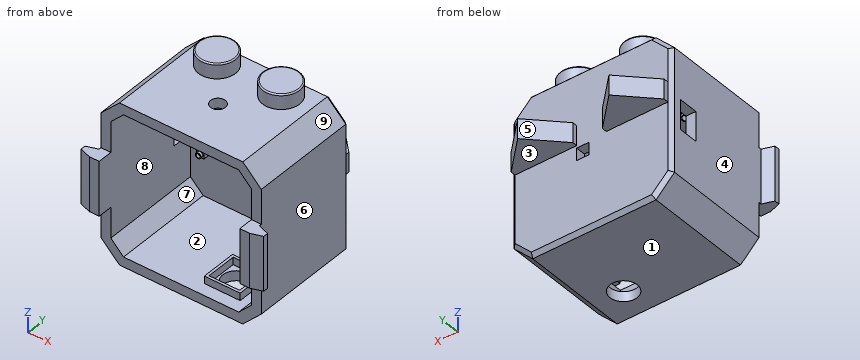
from build123d import *

# Parameters (mm, degrees)
SALIENTE_EXTRUIR1_DEPTH  = 45
VACIADO2_T               = -4
CHAFL_N3_SIZE            = 1.5
CROQUIS2_R               = 7.5
SALIENTE_EXTRUIR2_DEPTH  = 6
CROQUIS4_R               = 5
CORTAR_EXTRUIR2_DEPTH    = 8
REDONDEO1_R              = 0.5
CROQUIS5_R               = 3
CORTAR_EXTRUIR3_DEPTH    = 10
SALIENTE_EXTRUIR8_START  = 8
CROQUIS13_R              = 5
CROQUIS13_R_2            = 2.6
SALIENTE_EXTRUIR8_DEPTH  = 8
CROQUIS7_W               = 4
CROQUIS7_H               = 4
SALIENTE_EXTRUIR3_DEPTH  = 1
CROQUIS8_R               = 2
SALIENTE_EXTRUIR4_DEPTH  = 1
CROQUIS9_R               = 1.6
CORTAR_EXTRUIR5_DEPTH    = 2
CROQUIS10_W              = 25
CROQUIS10_H              = 8
SALIENTE_EXTRUIR5_DEPTH  = 2
SALIENTE_EXTRUIR6_DEPTH  = 8
CROQUIS12_R              = 1.15
CROQUIS12_R_2            = 0.8
SALIENTE_EXTRUIR7_DEPTH  = 6
CROQUIS14_W              = 3
CROQUIS14_H              = 2.5
SALIENTE_EXTRUIR9_DEPTH  = 5
CROQUIS15_W              = 12
CROQUIS15_H              = 8
CORTAR_EXTRUIR6_DEPTH    = 7
CROQUIS16_W              = 14.5
CROQUIS16_H              = 14.5
CROQUIS16_W_2            = 12.4
CROQUIS16_H_2            = 12.4
SALIENTE_EXTRUIR10_DEPTH = 3
CROQUIS17_R              = 5.5
CORTAR_EXTRUIR7_DEPTH    = 96.317889192
CROQUIS18_W              = 4
CROQUIS18_H              = 22
SALIENTE_EXTRUIR11_DEPTH = 6
SALIENTE_EXTRUIR13_DEPTH = 22
CROQUIS20_W              = 5
CROQUIS20_H              = 5
CORTAR_EXTRUIR8_DEPTH    = 10


with BuildPart() as part:
    # Croquis1 → Saliente-Extruir1 (new body)
    with BuildSketch(Plane(origin=(0, 0, 0), x_dir=(1, 0, 0), z_dir=(0, 1, 0))):
        Polygon((-25, -32.5), (25, -32.5), (32.5, -25), (32.5, 25), (25, 32.5), (-25, 32.5), (-32.5, 25), (-32.5, -25), align=None)
    extrude(amount=SALIENTE_EXTRUIR1_DEPTH)

    # Vaciado2
    vaciado2_openings = [part.faces().sort_by_distance(p)[0] for p in [
        (0, 0, 0),
    ]]
    offset(amount=VACIADO2_T, openings=vaciado2_openings, kind=Kind.INTERSECTION)

    # Chaflán3
    chafl_n3_edges = [part.edges().sort_by_distance(p)[0] for p in [
        (-28.75, 45, -28.75),
        (-32.5, 45, 0),
        (-28.75, 45, 28.75),
        (0, 45, 32.5),
        (28.75, 45, 28.75),
        (32.5, 45, 0),
        (28.75, 45, -28.75),
        (0, 45, -32.5),
    ]]
    chamfer(chafl_n3_edges, length=CHAFL_N3_SIZE)

    # Croquis2 → Saliente-Extruir2 (add)
    with BuildSketch(Plane.XY.offset(32.5)):
        with Locations(Location((13, 35, 0), (0, 0, 180))):
            Circle(CROQUIS2_R)
        with Locations(Location((-13, 35, 0), (0, 0, 180))):
            Circle(CROQUIS2_R)
    extrude(amount=SALIENTE_EXTRUIR2_DEPTH)

    # Croquis4 → Cortar-Extruir2 (cut)
    with BuildSketch(Plane(origin=(0, 0, 28.5), x_dir=(-1, 0, 0), z_dir=(0, 0, -1))):
        with Locations((-13, 35)):
            Circle(CROQUIS4_R)
        with Locations(Location((13, 35, 0), (0, 0, 180))):
            Circle(CROQUIS4_R)
    extrude(amount=-CORTAR_EXTRUIR2_DEPTH, mode=Mode.SUBTRACT)

    # Redondeo1
    redondeo1_edges = [part.edges().sort_by_distance(p)[0] for p in [
        (20.5, 35, 38.5),
        (-5.5, 35, 38.5),
    ]]
    fillet(redondeo1_edges, radius=REDONDEO1_R)

    # Croquis5 → Cortar-Extruir3 (cut)
    with BuildSketch(Plane.XY.offset(32.5)):
        with Locations((0, 19)):
            Circle(CROQUIS5_R)
    extrude(amount=-CORTAR_EXTRUIR3_DEPTH, mode=Mode.SUBTRACT)

    # Croquis13 → Saliente-Extruir8 (add)
    # profile 1 of 2: a face of its own
    with BuildSketch(Plane(origin=(0, 0, 36.5), x_dir=(-1, 0, 0), z_dir=(0, 0, -1)).offset(SALIENTE_EXTRUIR8_START)):
        with Locations((13, 35)):
            Circle(CROQUIS13_R)
        with Locations((13, 35)):
            Circle(CROQUIS13_R_2, mode=Mode.SUBTRACT)
    # profile 2 of 2: a face of its own
    with BuildSketch(Plane(origin=(0, 0, 36.5), x_dir=(-1, 0, 0), z_dir=(0, 0, -1)).offset(SALIENTE_EXTRUIR8_START)):
        with Locations((-13, 35)):
            Circle(CROQUIS13_R)
        with Locations((-13, 35)):
            Circle(CROQUIS13_R_2, mode=Mode.SUBTRACT)
    extrude(amount=-SALIENTE_EXTRUIR8_DEPTH)

    # Croquis7 → Saliente-Extruir3 (add)
    with BuildSketch(Plane(origin=(0, 0, 28.5), x_dir=(-1, 0, 0), z_dir=(0, 0, -1))):
        with Locations((-11.58, 10.5)):
            Rectangle(CROQUIS7_W, CROQUIS7_H)
        with Locations((-11.58, 28)):
            Rectangle(CROQUIS7_W, CROQUIS7_H)
        with Locations((11.43, 10.5)):
            Rectangle(CROQUIS7_W, CROQUIS7_H)
        with Locations((11.43, 28)):
            Rectangle(CROQUIS7_W, CROQUIS7_H)
    extrude(amount=SALIENTE_EXTRUIR3_DEPTH)

    # Croquis8 → Saliente-Extruir4 (add)
    with BuildSketch(Plane(origin=(0, 0, 27.5), x_dir=(-1, 0, 0), z_dir=(0, 0, -1))):
        with Locations(Location((-11.505, 10.489346828, 0), (0, 0, 264.083633631))):
            Circle(CROQUIS8_R)
        with Locations(Location((-11.505, 27.976317365, 0), (0, 0, 261.173934846))):
            Circle(CROQUIS8_R)
        with Locations(Location((11.505, 10.489346828, 0), (0, 0, 180))):
            Circle(CROQUIS8_R)
        with Locations(Location((11.505, 27.976317365, 0), (0, 0, 180))):
            Circle(CROQUIS8_R)
    extrude(amount=SALIENTE_EXTRUIR4_DEPTH)

    # Croquis9 → Cortar-Extruir5 (cut)
    with BuildSketch(Plane(origin=(0, 0, 26.5), x_dir=(-1, 0, 0), z_dir=(0, 0, -1))):
        with Locations((-11.505, 27.976317365)):
            Circle(CROQUIS9_R)
        with Locations((-11.505, 10.489346828)):
            Circle(CROQUIS9_R)
        with Locations((11.505, 10.489346828)):
            Circle(CROQUIS9_R)
        with Locations((11.505, 27.976317365)):
            Circle(CROQUIS9_R)
    extrude(amount=-CORTAR_EXTRUIR5_DEPTH, mode=Mode.SUBTRACT)

    # Croquis10 → Saliente-Extruir5 (add)
    with BuildSketch(Plane(origin=(0, 45, 0), x_dir=(1, 0, 0), z_dir=(0, 1, 0))):
        with Locations((-18.5, -7)):
            Rectangle(CROQUIS10_W, CROQUIS10_H)
        with Locations((18.5, -7)):
            Rectangle(CROQUIS10_W, CROQUIS10_H)
    extrude(amount=SALIENTE_EXTRUIR5_DEPTH)

    # Croquis11 → Saliente-Extruir6 (add)
    with BuildSketch(Plane.XY.offset(11)):
        Polygon((-31, 47), (-6, 47), (-18.5, 59.5), align=None)
        Polygon((31, 47), (18.5, 59.5), (6, 47), align=None)
    extrude(amount=-SALIENTE_EXTRUIR6_DEPTH)

    # Croquis12 → Saliente-Extruir7 (add)
    # profile 1 of 4: a face of its own
    with BuildSketch(Plane.XZ.offset(-41)):
        with Locations(Location((-20.65, 7.68, 0), (0, 0, 270))):
            Circle(CROQUIS12_R)
        with Locations(Location((-20.65, 7.68, 0), (0, 0, 270))):
            Circle(CROQUIS12_R_2, mode=Mode.SUBTRACT)
    # profile 2 of 4: a face of its own
    with BuildSketch(Plane.XZ.offset(-41)):
        with Locations(Location((-20.65, -7.68, 0), (0, 0, 90))):
            Circle(CROQUIS12_R)
        with Locations(Location((-20.65, -7.68, 0), (0, 0, 90))):
            Circle(CROQUIS12_R_2, mode=Mode.SUBTRACT)
    # profile 3 of 4: a face of its own
    with BuildSketch(Plane.XZ.offset(-41)):
        with Locations(Location((20.65, 7.68, 0), (0, 0, 90))):
            Circle(CROQUIS12_R)
        with Locations(Location((20.65, 7.68, 0), (0, 0, 90))):
            Circle(CROQUIS12_R_2, mode=Mode.SUBTRACT)
    # profile 4 of 4: a face of its own
    with BuildSketch(Plane.XZ.offset(-41)):
        with Locations(Location((20.65, -7.68, 0), (0, 0, 270))):
            Circle(CROQUIS12_R)
        with Locations(Location((20.65, -7.68, 0), (0, 0, 270))):
            Circle(CROQUIS12_R_2, mode=Mode.SUBTRACT)
    extrude(amount=SALIENTE_EXTRUIR7_DEPTH)

    # Croquis14 → Saliente-Extruir9 (add)
    with BuildSketch(Plane.XZ.offset(-41)):
        with Locations((-20.65, 7.68)):
            Rectangle(CROQUIS14_W, CROQUIS14_H)
        with Locations((-20.65, -7.68)):
            Rectangle(CROQUIS14_W, CROQUIS14_H)
        with Locations((20.65, 7.68)):
            Rectangle(CROQUIS14_W, CROQUIS14_H)
        with Locations((20.65, -7.68)):
            Rectangle(CROQUIS14_W, CROQUIS14_H)
    extrude(amount=SALIENTE_EXTRUIR9_DEPTH)

    # Croquis15 → Cortar-Extruir6 (cut)
    with BuildSketch(Plane.ZY.offset(32.5)):
        with Locations((0, 36.5)):
            Rectangle(CROQUIS15_W, CROQUIS15_H)
    extrude(amount=-CORTAR_EXTRUIR6_DEPTH, mode=Mode.SUBTRACT)

    # Croquis16 → Saliente-Extruir10 (add)
    with BuildSketch(Plane.XY.offset(-28.5)):
        with Locations((12.75, 12.25)):
            Rectangle(CROQUIS16_W, CROQUIS16_H)
        with Locations((12.75, 12.25)):
            Rectangle(CROQUIS16_W_2, CROQUIS16_H_2, mode=Mode.SUBTRACT)
    extrude(amount=SALIENTE_EXTRUIR10_DEPTH)

    # Croquis17 → Cortar-Extruir7 (cut, through all)
    with BuildSketch(Plane.XY.offset(-28.5)):
        with Locations((12.75, 12.25)):
            Circle(CROQUIS17_R)
    extrude(amount=-CORTAR_EXTRUIR7_DEPTH, mode=Mode.SUBTRACT)

    # Croquis18 → Saliente-Extruir11 (add)
    with BuildSketch(Plane.XZ):
        with Locations((-30.5, 0)):
            Rectangle(CROQUIS18_W, CROQUIS18_H)
        with Locations((30.5, 0)):
            Rectangle(CROQUIS18_W, CROQUIS18_H)
    extrude(amount=SALIENTE_EXTRUIR11_DEPTH)

    # Croquis19 → Saliente-Extruir13 (add)
    with BuildSketch(Plane.XY.offset(11)):
        Polygon((-32.5, -1), (-37, -2.5), (-37, -4.5), (-32.5, -6), align=None)
        Polygon((37, -2.5), (37, -4.5), (32.5, -6), (32.5, -1), align=None)
    extrude(amount=-SALIENTE_EXTRUIR13_DEPTH)

    # Croquis20 → Cortar-Extruir8 (cut)
    with BuildSketch(Plane(origin=(0, 45, 0), x_dir=(1, 0, 0), z_dir=(0, 1, 0))):
        with Locations((3.50287975, 0.5)):
            Rectangle(CROQUIS20_W, CROQUIS20_H)
    extrude(amount=-CORTAR_EXTRUIR8_DEPTH, mode=Mode.SUBTRACT)


solid = part.part
The listing builds one solid part. Answer for the finished solid, in the listing's coordinates (mm). Face numbers are marked on the shaded views. A direction names the side the tool comes from. Round coordinates to 2 decimals unless told otherwise and drop trailing zeros. Write each loop counter-clockwise with the first axis right and the second up, starting at its lowest first coordinate (ties: lowest second). Pieces come first, ordered by that corner, then holes. Notation, with made-up numbers: M 76,-27 L 121,-27 A30 cw 121,2 Z; hole C -36.75,-37 d8. An arc over 180 degrees is marked long. Write each question's results on one line, items separated by ' | '. Start each with the question number.
Item 1: A cutting plane is placed at C-C on y = 13.5. Write down the section's boundary in (x, z).
Item 2: Straight lines are drawn through the part: L1, parallel to Z at x = -21, y = 22.5; L2, parallel to Z at x = 5, y = 42.5. For each, find the intervals that lie inside material, in ascending order. Write a range as [from, to].
Item 3: For a pull along Z with two mould halves and no side action, classify the marked faces 6, 7, 8 and 9 as pulls with the +Z half, pulls with the -Z half, needs draft (parallel to the pull), parting line crosses it, or undercut.
Item 4: A cutting plane is placed at D-D on y = 39.5. State how many separate pieces and enclosed holes the cut face has, and give its area (3 significant figures).
Item 5: Flat-ended cylindrical pins translate along their axes: pin 1 Ø6 at (x, y) = (10.5, 20.5) entering from +Z; pin 2 Ø3 at (y, z) = (39, -8.5) entering from +X; pin 3 Ø0.6 at (y, z) = (45.5, 9) entering from -X. Find the tip coordinate at first contact, or state that the pin passes through.
Item 6: For the marked faces 1, 2, 3, 4 and 5, determine the directions among +Z, -Z, +X, -X, +Y, -Y from which every point of the face is accessible in a straight line to the end or side of a thin tool.
Item 7: A cutting plane is placed at A-A on y = 55. Write down the section's boundary in (x, z), and give its area (3 significant figures).
Item 8: A cutting plane is placed at B-B on z = 10. Write down the section's boundary in (x, y).
Check sheet entries:
1) outline: M -32.5,-25 L -25,-32.5 L 7.39,-32.5 L 7.39,-28.5 L 6.55,-28.5 L 6.55,-25.5 L 5.5,-25.5 L 5.5,-28.5 L -23.34,-28.5 L -28.5,-23.34 L -28.5,23.34 L -23.34,28.5 L 23.34,28.5 L 28.5,23.34 L 28.5,-23.34 L 23.34,-28.5 L 20,-28.5 L 20,-25.5 L 18.95,-25.5 L 18.95,-28.5 L 18.11,-28.5 L 18.11,-32.5 L 25,-32.5 L 32.5,-25 L 32.5,25 L 25,32.5 L -25,32.5 L -32.5,25 Z
2) L1: [-32.5, -28.5], [28.5, 32.5] | L2: [-32.5, -3], [2, 32.5]
3) face 6: needs draft | face 7: undercut | face 8: undercut | face 9: pulls with the +Z half
4) separate pieces: 5 | enclosed holes: 0 | area: 1,040 mm²
5) pin 1: z = 32.5 | pin 2: x = 32.5 | pin 3: x = -31
6) face 1: -Z, +X, -X, +Y, -Y | face 2: none | face 3: -Z, +X, -X, +Y | face 4: +Z, -Z, -X, +Y | face 5: +Z, -Z, +Y
7) outline: M -23,3 L -14,3 L -14,11 L -23,11 Z; M 14,3 L 23,3 L 23,11 L 14,11 Z | area: 144 mm²
8) outline: M -37,-4.5 L -32.5,-6 L -28.5,-6 L -28.5,41 L 28.5,41 L 28.5,-6 L 32.5,-6 L 37,-4.5 L 37,-2.5 L 32.5,-1 L 32.5,43.5 L 31,45 L 31,47 L 18.5,59.5 L 6,47 L 6,45 L -6,45 L -6,47 L -18.5,59.5 L -31,47 L -31,45 L -32.5,43.5 L -32.5,-1 L -37,-2.5 Z
